```python
from build123d import *

# Parameters (mm, degrees)
SKETCH1_R           = 7.9
BOSS_EXTRUDE1_DEPTH = 3
SKETCH3_W           = 5
SKETCH3_H           = 150
CUT_EXTRUDE2_DEPTH  = 213.888468452
FILLET2_R           = 2.5
SKETCH4_W           = 5
SKETCH4_H           = 2
BOSS_EXTRUDE2_DEPTH = 3
FILLET3_R           = 2.5


with BuildPart() as part:
    # Sketch1 → Boss-Extrude1 (new body)
    with BuildSketch(Plane(origin=(0, 0, 0), x_dir=(0, 0, -1), z_dir=(1, 0, 0))):
        with BuildLine():
            Line((7.5, 10), (7.5, 190))
            ThreePointArc((7.5, 190), (0, 212.5), (-7.5, 190))
            Line((-7.5, 190), (-7.5, 10))
            ThreePointArc((-7.5, 10), (0, -12.5), (7.5, 10))
        make_face()
        Circle(SKETCH1_R, mode=Mode.SUBTRACT)
        with Locations((0, 200)):
            Circle(SKETCH1_R, mode=Mode.SUBTRACT)
    extrude(amount=BOSS_EXTRUDE1_DEPTH)

    # Sketch3 → Cut-Extrude2 (cut, through all)
    with BuildSketch(Plane(origin=(3, 0, 0), x_dir=(0, 0, -1), z_dir=(1, 0, 0))):
        with Locations((0, 100)):
            Rectangle(SKETCH3_W, SKETCH3_H)
    extrude(amount=-CUT_EXTRUDE2_DEPTH, mode=Mode.SUBTRACT)

    # Fillet2
    fillet2_edges = [part.edges().sort_by_distance(p)[0] for p in [
        (1.5, 175, 2.5),
        (1.5, 175, -2.5),
        (1.5, 25, 2.5),
        (1.5, 25, -2.5),
    ]]
    fillet(fillet2_edges, radius=FILLET2_R - 0.0001)  # a hair under: the kernel refuses the full size

    # Sketch4 → Boss-Extrude2 (add)
    with BuildSketch(Plane(origin=(3, 0, 0), x_dir=(0, 0, -1), z_dir=(1, 0, 0))):
        with Locations((0, 100.007044109)):
            Rectangle(SKETCH4_W, SKETCH4_H)
        with Locations((0, 50.007044109)):
            Rectangle(SKETCH4_W, SKETCH4_H)
        with Locations((0, 150.007044109)):
            Rectangle(SKETCH4_W, SKETCH4_H)
    extrude(amount=-BOSS_EXTRUDE2_DEPTH)

    # Fillet3
    fillet3_edges = [part.edges().sort_by_distance(p)[0] for p in [
        (1.5, 101.007044109, -2.5),
        (1.5, 101.007044109, 2.5),
        (1.5, 51.007044109, 2.5),
        (1.5, 51.007044109, -2.5),
        (1.5, 49.007044109, 2.5),
        (1.5, 49.007044109, -2.5),
        (1.5, 99.007044109, -2.5),
        (1.5, 99.007044109, 2.5),
        (1.5, 149.007044109, 2.5),
        (1.5, 149.007044109, -2.5),
        (1.5, 151.007044109, 2.5),
        (1.5, 151.007044109, -2.5),
    ]]
    fillet(fillet3_edges, radius=FILLET3_R - 0.0001)  # a hair under: the kernel refuses the full size


solid = part.part
```
Read the model definition and answer for the solid it produces. Units are mm, in the model's axes. Round coordinates to 2 decimals unless told otherwise and drop trailing zeros. Write each loop counter-clockwise with the first axis right and the second up, starting at its lowest first coordinate (ties: lowest second). Pieces come first, ordered by that corner, then holes. Notation, with made-up numbers: (-39.5, 11.5) -> (-22.5, 11.5) arc R28 ccw to (-22.5, 46.5) -> close; hole circle Ø3 at (74, -27). An arc over 180 degrees is marked (long way). Answer in a Markdown table with one row per item. Add a question column.
1) Consider line 1 (Y direction, x = 2.6, z = 3.75); line 2 (Z direction, x = 2.8, y = 75); line 3 (Y direction, x = 1.95, z = -6). Determine where each line is inside the solid, lowest interval first.
2) Find section A-A, the plane y = 120.5. Determine the outline of the cut face in (x, z), and give its area (3 significant figures).
3) Given P1, Ø1.5, axis at x = 1, y = 133.5, coming from the -Z side; P2, Ø6, axis at y = 149.5, z = 8.5, coming from the -X side; P3, Ø0.9, axis at x = 2, y = 167, coming from the +Z side, each flat-ended and moving along its own axis, determine where each tip first touches the part or whether it passes through.
4) Find section B-B, the plane y = 200. Determine the outline of the cut face in (x, z), and give its area (3 significant figures).
Findings below:
| question | item | result |
|---|---|---|
| 1 | line 1 | -11.92 to -6.95, 6.95 to 193.05, 206.95 to 211.92 |
| 1 | line 2 | -7.5 to -2.5, 2.5 to 7.5 |
| 1 | line 3 | -10.97 to -5.14, 5.14 to 194.86, 205.14 to 210.97 |
| 2 | outline | (0, -7.5) -> (3, -7.5) -> (3, -2.5) -> (0, -2.5) -> close; (0, 2.5) -> (3, 2.5) -> (3, 7.5) -> (0, 7.5) -> close |
| 2 | area | 30.0 mm² |
| 3 | P1 | z = -7.5 |
| 3 | P2 | x = 0 |
| 3 | P3 | z = 7.5 |
| 4 | outline | (0, -12.5) -> (3, -12.5) -> (3, -7.9) -> (0, -7.9) -> close; (0, 7.9) -> (3, 7.9) -> (3, 12.5) -> (0, 12.5) -> close |
| 4 | area | 27.6 mm² |
